from build123d import *

# Parameters (mm, degrees)
SKETCH1_W                      = 175
SKETCH1_H                      = 100
BOSS_EXTRUDE1_DEPTH            = 1.9
CUT_EXTRUDE1_REACH             = 102.796
SKETCH2_R                      = 1.8288
CUT_EXTRUDE1_DIRECTION_2_DEPTH = 101.796130878
FILLET1_R                      = 3.175
CUT_EXTRUDE2_REACH             = 102.796
SKETCH3_R                      = 1.65
SKETCH3_R_2                    = 2.0193


with BuildPart() as part:
    # Sketch1 → Boss-Extrude1 (new body)
    with BuildSketch(Plane.XY):
        Rectangle(SKETCH1_W, SKETCH1_H)
    extrude(amount=BOSS_EXTRUDE1_DEPTH)

    # Sketch2 → Cut-Extrude1 (cut, up to next)
    with BuildSketch(Plane(origin=(0, 0, 0), x_dir=(-1, 0, 0), z_dir=(0, 0, -1)), mode=Mode.PRIVATE) as cut_extrude1_sk1:
        with Locations(Location((-81.15, 43.65, 0), (0, 0, 180))):
            Circle(SKETCH2_R)
    cut_extrude1_tool1 = extrude(cut_extrude1_sk1.sketch, amount=-CUT_EXTRUDE1_REACH, mode=Mode.PRIVATE) & part.part
    # Sketch2 → Cut-Extrude1 (cut, up to next)
    with BuildSketch(Plane(origin=(0, 0, 0), x_dir=(-1, 0, 0), z_dir=(0, 0, -1)), mode=Mode.PRIVATE) as cut_extrude1_sk2:
        with Locations(Location((-81.15, -43.65, 0), (0, 0, 180))):
            Circle(SKETCH2_R)
    cut_extrude1_tool2 = extrude(cut_extrude1_sk2.sketch, amount=-CUT_EXTRUDE1_REACH, mode=Mode.PRIVATE) & part.part
    # Sketch2 → Cut-Extrude1 (cut, up to next)
    with BuildSketch(Plane(origin=(0, 0, 0), x_dir=(-1, 0, 0), z_dir=(0, 0, -1)), mode=Mode.PRIVATE) as cut_extrude1_sk3:
        with Locations(Location((81.15, 43.65, 0), (0, 0, 180))):
            Circle(SKETCH2_R)
    cut_extrude1_tool3 = extrude(cut_extrude1_sk3.sketch, amount=-CUT_EXTRUDE1_REACH, mode=Mode.PRIVATE) & part.part
    # Sketch2 → Cut-Extrude1 (cut, up to next)
    with BuildSketch(Plane(origin=(0, 0, 0), x_dir=(-1, 0, 0), z_dir=(0, 0, -1)), mode=Mode.PRIVATE) as cut_extrude1_sk4:
        with Locations(Location((81.15, -43.65, 0), (0, 0, 180))):
            Circle(SKETCH2_R)
    cut_extrude1_tool4 = extrude(cut_extrude1_sk4.sketch, amount=-CUT_EXTRUDE1_REACH, mode=Mode.PRIVATE) & part.part
    add(cut_extrude1_tool1.solids().sort_by_distance((81.15, 43.65, 0))[0], mode=Mode.SUBTRACT)
    add(cut_extrude1_tool2.solids().sort_by_distance((81.15, -43.65, 0))[0], mode=Mode.SUBTRACT)
    add(cut_extrude1_tool3.solids().sort_by_distance((-81.15, 43.65, 0))[0], mode=Mode.SUBTRACT)
    add(cut_extrude1_tool4.solids().sort_by_distance((-81.15, -43.65, 0))[0], mode=Mode.SUBTRACT)

    # Sketch2 → Cut-Extrude1 direction 2 (cut)
    with BuildSketch(Plane(origin=(0, 0, 0), x_dir=(-1, 0, 0), z_dir=(0, 0, -1))):
        with Locations(Location((-81.15, 43.65, 0), (0, 0, 180))):
            Circle(SKETCH2_R)
        with Locations(Location((-81.15, -43.65, 0), (0, 0, 180))):
            Circle(SKETCH2_R)
        with Locations(Location((81.15, 43.65, 0), (0, 0, 180))):
            Circle(SKETCH2_R)
        with Locations(Location((81.15, -43.65, 0), (0, 0, 180))):
            Circle(SKETCH2_R)
    extrude(amount=CUT_EXTRUDE1_DIRECTION_2_DEPTH, mode=Mode.SUBTRACT)

    # Fillet1
    fillet1_edges = [part.edges().sort_by_distance(p)[0] for p in [
        (87.5, -50, 0.95),
        (-87.5, -50, 0.95),
        (-87.5, 50, 0.95),
        (87.5, 50, 0.95),
    ]]
    fillet(fillet1_edges, radius=FILLET1_R)

    # Sketch3 → Cut-Extrude2 (cut, up to next)
    with BuildSketch(Plane.XY.offset(1.9), mode=Mode.PRIVATE) as cut_extrude2_sk1:
        with Locations((-49.1, -19.85)):
            Circle(SKETCH3_R)
    cut_extrude2_tool1 = extrude(cut_extrude2_sk1.sketch, amount=-CUT_EXTRUDE2_REACH, mode=Mode.PRIVATE) & part.part
    # Sketch3 → Cut-Extrude2 (cut, up to next)
    with BuildSketch(Plane.XY.offset(1.9), mode=Mode.PRIVATE) as cut_extrude2_sk2:
        with Locations((-70.5, 19.85)):
            Circle(SKETCH3_R)
    cut_extrude2_tool2 = extrude(cut_extrude2_sk2.sketch, amount=-CUT_EXTRUDE2_REACH, mode=Mode.PRIVATE) & part.part
    # Sketch3 → Cut-Extrude2 (cut, up to next)
    with BuildSketch(Plane.XY.offset(1.9), mode=Mode.PRIVATE) as cut_extrude2_sk3:
        with Locations((6.3, -19.85)):
            Circle(SKETCH3_R)
    cut_extrude2_tool3 = extrude(cut_extrude2_sk3.sketch, amount=-CUT_EXTRUDE2_REACH, mode=Mode.PRIVATE) & part.part
    # Sketch3 → Cut-Extrude2 (cut, up to next)
    with BuildSketch(Plane.XY.offset(1.9), mode=Mode.PRIVATE) as cut_extrude2_sk4:
        with Locations((-15.1, 19.85)):
            Circle(SKETCH3_R)
    cut_extrude2_tool4 = extrude(cut_extrude2_sk4.sketch, amount=-CUT_EXTRUDE2_REACH, mode=Mode.PRIVATE) & part.part
    # Sketch3 → Cut-Extrude2 (cut, up to next)
    with BuildSketch(Plane.XY.offset(1.9), mode=Mode.PRIVATE) as cut_extrude2_sk5:
        with Locations((58.29, -31.115)):
            Circle(SKETCH3_R_2)
    cut_extrude2_tool5 = extrude(cut_extrude2_sk5.sketch, amount=-CUT_EXTRUDE2_REACH, mode=Mode.PRIVATE) & part.part
    # Sketch3 → Cut-Extrude2 (cut, up to next)
    with BuildSketch(Plane.XY.offset(1.9), mode=Mode.PRIVATE) as cut_extrude2_sk6:
        with Locations((58.29, 31.115)):
            Circle(SKETCH3_R_2)
    cut_extrude2_tool6 = extrude(cut_extrude2_sk6.sketch, amount=-CUT_EXTRUDE2_REACH, mode=Mode.PRIVATE) & part.part
    add(cut_extrude2_tool1.solids().sort_by_distance((-49.1, -19.85, 1.9))[0], mode=Mode.SUBTRACT)
    add(cut_extrude2_tool2.solids().sort_by_distance((-70.5, 19.85, 1.9))[0], mode=Mode.SUBTRACT)
    add(cut_extrude2_tool3.solids().sort_by_distance((6.3, -19.85, 1.9))[0], mode=Mode.SUBTRACT)
    add(cut_extrude2_tool4.solids().sort_by_distance((-15.1, 19.85, 1.9))[0], mode=Mode.SUBTRACT)
    add(cut_extrude2_tool5.solids().sort_by_distance((58.29, -31.115, 1.9))[0], mode=Mode.SUBTRACT)
    add(cut_extrude2_tool6.solids().sort_by_distance((58.29, 31.115, 1.9))[0], mode=Mode.SUBTRACT)


solid = part.part
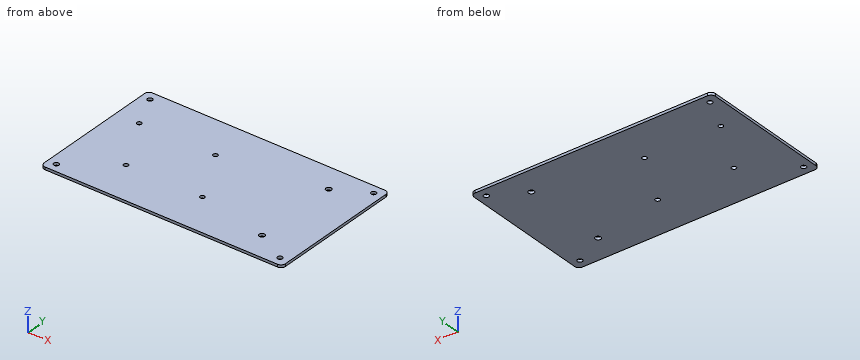
Geometry: final body of the model. Coordinates: model frame, mm. Give positions to 0.01 mm unless a question says otherwise; leave off trailing zeros. Loops run counter-clockwise (first coordinate to the right, second up) from the corner with the lowest first, then second, coordinate; pieces in that order, holes last. Notation, with made-up numbers: (72.5, -33.75) - (92.5, -33.75) arc R17 cw to (92.5, -16.75) - close; hole circle Ø2 at (69, 23.25). An arc over 180 degrees is marked (long way). One line per question, with ' | ' between items. Start each with the question number.
(1) Ray query, line 1 (Y direction, x = -81.15, z = 1.2); line 2 (X direction, y = -43.65, z = 0.55); line 3 (Y direction, x = 6.3, z = 1). Return the intervals inside material, ascending. Write a range as from..to.
(2) Section query B-B on x = 81.15. Return loops of the section in (y, z), then the cut area to 3 significant figures.
(3) Section query C-C on y = -43.65. Return loops of the section in (x, z), then the cut area to 3 significant figures.
(4) Section query A-A on x = -49.1. Return loops of the section in (y, z), then the cut area to 3 significant figures.
The answers:
1) line 1: -50..-45.48, -41.82..41.82, 45.48..50 | line 2: -87.5..-82.98, -79.32..79.32, 82.98..87.5 | line 3: -50..-21.5, -18.2..50
2) outline: (-50, 0) - (-45.48, 0) - (-45.48, 1.9) - (-50, 1.9) - close; (-41.82, 0) - (41.82, 0) - (41.82, 1.9) - (-41.82, 1.9) - close; (45.48, 0) - (50, 0) - (50, 1.9) - (45.48, 1.9) - close | area: 176 mm2
3) outline: (-87.5, 0) - (-82.98, 0) - (-82.98, 1.9) - (-87.5, 1.9) - close; (-79.32, 0) - (79.32, 0) - (79.32, 1.9) - (-79.32, 1.9) - close; (82.98, 0) - (87.5, 0) - (87.5, 1.9) - (82.98, 1.9) - close | area: 319 mm2
4) outline: (-50, 0) - (-21.5, 0) - (-21.5, 1.9) - (-50, 1.9) - close; (-18.2, 0) - (50, 0) - (50, 1.9) - (-18.2, 1.9) - close | area: 184 mm2
